Can you work these out from the model? Positions are in its coordinate system, mm. Face numbers are marked on the shaded views. A direction names the side the tool comes from. Give positions to 0.01 mm unless a question says otherwise; leave off trailing zeros. Write each loop counter-clockwise with the first axis right and the second up, starting at its lowest first coordinate (ties: lowest second). Pieces come first, ordered by that corner, then holes. Notation, with made-up numbers: M -5.75,54 L 30.25,54 A19 ccw 30.25,63 Z; hole C -14,33.5 d2. An arc over 180 degrees is marked long. Write each question's results on one line, items separated by ' | '.
from build123d import *

# Parameters (mm, degrees)
BOSS_EXTRUDE1_DEPTH      = 100
FILLET1_R                = 30
FILLET2_R                = 17
BOSS_EXTRUDE2_DEPTH      = 17
BOSS_EXTRUDE2_DEPTH_BACK = 13
CUT_EXTRUDE1_START       = -17
SKETCH2_4_W              = 100
SKETCH2_4_H              = 30.125527048
CUT_EXTRUDE1_DEPTH       = 17
FILLET3_R                = 50
BOSS_EXTRUDE3_DEPTH      = 5
BOSS_EXTRUDE3_DEPTH_BACK = 18
SKETCH3_R                = 30
SKETCH3_R_2              = 20
SKETCH3_2_R              = 20
CUT_EXTRUDE2_DEPTH       = 25
CUT_EXTRUDE3_DEPTH       = 25
CUT_EXTRUDE4_DEPTH       = 25
CUT_EXTRUDE5_START       = -25
CUT_EXTRUDE5_DEPTH       = 25


with BuildPart() as part:
    # Sketch1 → Boss-Extrude1 (new body)
    with BuildSketch(Plane(origin=(0, 0, 0), x_dir=(0, 0, -1), z_dir=(1, 0, 0))):
        Polygon((0, 0), (0, 137), (144, 137), (144, 0), (157, 0), (157, 150), (-13, 150), (-13, 0), align=None)
    extrude(amount=BOSS_EXTRUDE1_DEPTH)

    # Fillet1
    fillet1_edges = [part.edges().sort_by_distance(p)[0] for p in [
        (50, 150, -157),
        (50, 150, 13),
    ]]
    fillet(fillet1_edges, radius=FILLET1_R)

    # Fillet2
    fillet2_edges = [part.edges().sort_by_distance(p)[0] for p in [
        (50, 137, 0),
        (50, 137, -144),
    ]]
    fillet(fillet2_edges, radius=FILLET2_R)

    # Sketch2 → Boss-Extrude2 (add, two sides: drawn at the far end of the back side and taken through both)
    with BuildSketch(Plane.XY.offset(13).offset(-BOSS_EXTRUDE2_DEPTH_BACK)):
        with BuildLine():
            Line((-12.5, 64), (112.5, 64))
            ThreePointArc((112.5, 64), (144.5, 32), (112.5, 0))
            Line((112.5, 0), (-12.5, 0))
            ThreePointArc((-12.5, 0), (-44.5, 32), (-12.5, 64))
        make_face()
        with BuildLine():
            Line((-12.5, 47.062763524), (112.5, 47.062763524))
            ThreePointArc((112.5, 47.062763524), (127.562763524, 32), (112.5, 16.937236476))
            Line((112.5, 16.937236476), (-12.5, 16.937236476))
            ThreePointArc((-12.5, 16.937236476), (-27.562763524, 32), (-12.5, 47.062763524))
        make_face(mode=Mode.SUBTRACT)
    extrude(amount=BOSS_EXTRUDE2_DEPTH + BOSS_EXTRUDE2_DEPTH_BACK)

    # Sketch2<4> → Cut-Extrude1 (cut)
    with BuildSketch(Plane.XY.offset(13).offset(CUT_EXTRUDE1_START)):
        with BuildLine():
            Line((0, 16.937236476), (0, 47.062763524))
            Line((0, 47.062763524), (-12.5, 47.062763524))
            ThreePointArc((-12.5, 47.062763524), (-27.562763524, 32), (-12.5, 16.937236476))
            Line((-12.5, 16.937236476), (0, 16.937236476))
        make_face()
        with Locations((50, 32)):
            Rectangle(SKETCH2_4_W, SKETCH2_4_H)
        with BuildLine():
            Line((112.5, 47.062763524), (100, 47.062763524))
            Line((100, 47.062763524), (100, 16.937236476))
            Line((100, 16.937236476), (112.5, 16.937236476))
            ThreePointArc((112.5, 16.937236476), (127.562763524, 32), (112.5, 47.062763524))
        make_face()
    extrude(amount=CUT_EXTRUDE1_DEPTH, mode=Mode.SUBTRACT)

    # Fillet3
    fillet3_edges = [part.edges().sort_by_distance(p)[0] for p in [
        (0, 0, -150.5),
        (100, 0, -150.5),
    ]]
    fillet(fillet3_edges, radius=FILLET3_R - 0.0001)  # a hair under: the kernel refuses the full size

    # Sketch3 → Boss-Extrude3 (add, two sides: drawn at the far end of the back side and taken through both)
    with BuildSketch(Plane(origin=(0, 0, -157), x_dir=(-1, 0, 0), z_dir=(0, 0, -1)).offset(-BOSS_EXTRUDE3_DEPTH_BACK)):
        with Locations(Location((-50, 50, 0), (0, 0, 90))):
            Circle(SKETCH3_R)
        with Locations(Location((-50, 50, 0), (0, 0, 90))):
            Circle(SKETCH3_R_2, mode=Mode.SUBTRACT)
    extrude(amount=BOSS_EXTRUDE3_DEPTH + BOSS_EXTRUDE3_DEPTH_BACK)

    # Sketch3<2> → Cut-Extrude2 (cut)
    with BuildSketch(Plane(origin=(0, 0, -157), x_dir=(-1, 0, 0), z_dir=(0, 0, -1))):
        with Locations(Location((-50, 50, 0), (0, 0, 90))):
            Circle(SKETCH3_2_R)
    extrude(amount=-CUT_EXTRUDE2_DEPTH, mode=Mode.SUBTRACT)

    # Sketch4 → Cut-Extrude3 (cut)
    with BuildSketch(Plane(origin=(0, 0, -157), x_dir=(-1, 0, 0), z_dir=(0, 0, -1))):
        with BuildLine():
            Line((-58, 150), (-58, 102))
            ThreePointArc((-58, 102), (-50, 94), (-42, 102))
            Line((-42, 102), (-42, 150))
            ThreePointArc((-42, 150), (-50, 158), (-58, 150))
        make_face()
    extrude(amount=-CUT_EXTRUDE3_DEPTH, mode=Mode.SUBTRACT)

    # Sketch5 → Cut-Extrude4 (cut)
    with BuildSketch(Plane(origin=(0, 150, 0), x_dir=(1, 0, 0), z_dir=(0, 1, 0))):
        with BuildLine():
            Line((58, 157), (58, 109))
            ThreePointArc((58, 109), (50, 101), (42, 109))
            Line((42, 109), (42, 157))
            ThreePointArc((42, 157), (50, 165), (58, 157))
        make_face()
        with BuildLine():
            Line((42, -13), (42, 35))
            ThreePointArc((42, 35), (50, 43), (58, 35))
            Line((58, 35), (58, -13))
            ThreePointArc((58, -13), (50, -21), (42, -13))
        make_face()
    extrude(amount=-CUT_EXTRUDE4_DEPTH, mode=Mode.SUBTRACT)

    # Sketch6 → Cut-Extrude5 (cut)
    with BuildSketch(Plane.XY.offset(13).offset(CUT_EXTRUDE5_START)):
        with BuildLine():
            Line((58, 150), (58, 102))
            ThreePointArc((58, 102), (50, 94), (42, 102))
            Line((42, 102), (42, 150))
            ThreePointArc((42, 150), (50, 158), (58, 150))
        make_face()
    extrude(amount=CUT_EXTRUDE5_DEPTH, mode=Mode.SUBTRACT)


solid = part.part
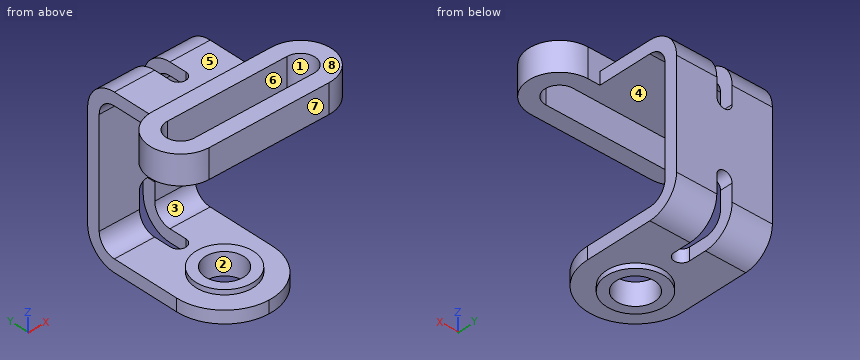
Item 1: I'm going to push flat-ended pins straight in: pin 1 (24 mm diameter, centred on y = 129.5, z = -126.5, fed in from +X); pin 2 (4 mm diameter, centred on x = 26, y = 131, fed in from +Z); pin 3 (5 mm diameter, centred on x = 42, z = -91, fed in from -Y). Where does each tip first touch, or does it pass through?
Geometry says:
pin 1: stops at x = 100 | pin 2: stops at z = 11.62 | pin 3: stops at y = 137
Item 2: I want a section at C-C, the plane y = 104.5. Please give me the cut outline in (x, z).
Geometry says:
outline: M 0,-157 L 42,-157 L 42,-144 L 0,-144 Z; M 0,0 L 42,0 L 42,13 L 0,13 Z; M 58,-157 L 100,-157 L 100,-144 L 58,-144 Z; M 58,0 L 100,0 L 100,13 L 58,13 Z
Item 3: Thinking about a two-plate mould opening in Y: for the marked faces 6, 7 and 8, which applies, +Y half, -Y half, draft (parallel to the pull), parting line (faces both ways), or undercut?
Geometry says:
face 6: undercut | face 7: -Y half | face 8: draft
Item 4: For the marked faces 1, 2, 3, 4 and 5, which set-ups out of +Z, -Z, +X, -X, +Y, -Y let a thin tool reach every point of the face, with its end or its side?
Geometry says:
face 1: +Z, -Z | face 2: -Z | face 3: +X, -X | face 4: +X, -X, -Y | face 5: +Z, +X, -X, +Y
Item 5: I want a section at D-D, the plane y = 56. Please give me the cut outline in (x, z), and give its area (3 significant figures).
Geometry says:
outline: M -33.67,0 L 133.67,0 L 133.67,30 L -33.67,30 Z; M 0,-157 L 20.61,-157 L 20.61,-162 L 30.92,-162 L 30.92,-139 L 20.61,-139 L 20.61,-144 L 0,-144 Z; M 69.08,-162 L 79.39,-162 L 79.39,-157 L 100,-157 L 100,-144 L 79.39,-144 L 79.39,-139 L 69.08,-139 Z | area: 6,030 mm2
Item 6: If I drill on line 1 (Z direction, x = 36, y = 75); line 2 (Z direction, x = 61.5, y = 84.5); line 3 (X direction, y = 50, z = -147), over which ranges is the centre line in solid material (lowest first)? Write a range as from..to.
Geometry says:
line 1: z = -162..-139, 0..13 | line 2: z = -157..-144, 0..13 | line 3: x = 0..30, 70..100
Item 7: I want a section at A-A, the plane x = -5. Please give me the cut outline in (y, z), and give its area (3 significant figures).
Geometry says:
outline: M 0,0 L 16.94,0 L 16.94,30 L 0,30 Z; M 47.06,0 L 64,0 L 64,30 L 47.06,30 Z | area: 1,020 mm2
Item 8: I want a section at B-B, the plane z = -124. Please give me the cut outline in (x, y).
Geometry says:
outline: M 0,137 L 42,137 L 42,150 L 0,150 Z; M 58,137 L 100,137 L 100,150 L 58,150 Z
